Source: CAD feature listing. Evaluate the final solid. Frame: model axes, mm. Coordinates: 2 decimals unless noted, no trailing zeros. Write each loop counter-clockwise with the first axis right and the second up, starting at its lowest first coordinate (ties: lowest second). Pieces come first, ordered by that corner, then holes. Notation, with made-up numbers: M -34,-12.5 L 8,-12.5 A34 cw 8,24.5 Z; hole C -29.75,82 d10. An arc over 180 degrees is marked long. One line per item, written item: value. Start each with the question number.
Item 1: Pin query (flat end, axial travel): P1, Ø8, axis at y = -8, z = 13.5, coming from the -X side; P2, Ø4, axis at x = 11.5, y = 9.5, coming from the +Z side; P3, Ø4, axis at y = 0, z = 33.5, coming from the +X side. Return the tip coordinate at first contact, or that it passes through.
Item 2: Cut plane A-A, the plane y = -1. Output: boundary loops of the cut face in (x, z) (1 decimal).
Item 3: Ray query, L1, parallel to Z at x = 35.5, y = 5; L2, parallel to X at y = -0.5, z = -10; L3, parallel to X at y = -11, z = 29. Return the intervals inside material, ascending. Write a range as from..to.
Item 4: Cut plane B-B, the plane y = 13.5. Output: boundary loops of the cut face in (x, z) (1 decimal), then the cut area to 3 significant figures.
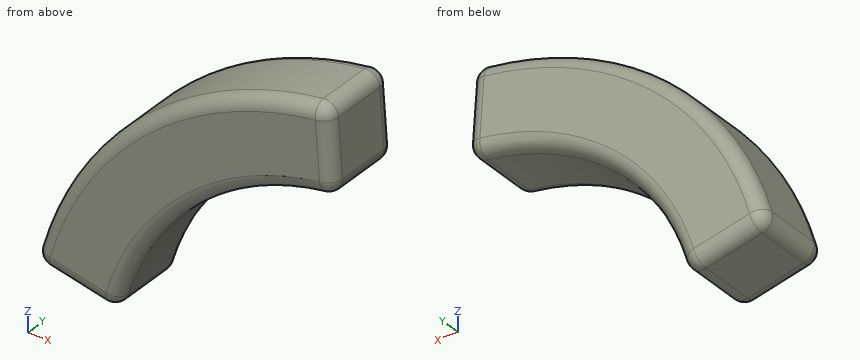
```python
from build123d import *

# Parameters (mm, degrees)
F1_DEPTH = 15.875
F2_R     = 5.08


with BuildPart() as f1:
    # F0 (on Front) → F1 (new body, symmetric)
    with BuildSketch(Plane.XZ):
        with BuildLine():
            ThreePointArc((-24.109727, -54.845564), (5.564563, -6.703762), (57.928178, 14.656209))
            Line((57.928178, 14.656209), (55.651654, 46.32449))
            ThreePointArc((55.651654, 46.32449), (-14.958741, 17.521359), (-54.973422, -47.396077))
            Line((-54.973422, -47.396077), (-24.109727, -54.845564))
        make_face()
    extrude(amount=F1_DEPTH, both=True)

    # F2
    f2_edges = [f1.edges().sort_by_distance(p)[0] for p in [
        (-14.958741, -15.875, 17.521359),
        (5.564563, -15.875, -6.703762),
        (57.928178, 0, 14.656209),
        (56.789916, 15.875, 30.490349),
        (55.651654, 0, 46.32449),
        (56.789916, -15.875, 30.490349),
        (-14.958741, 15.875, 17.521359),
        (5.564563, 15.875, -6.703762),
        (-24.109727, 0, -54.845564),
        (-39.541574, 15.875, -51.12082),
        (-54.973422, 0, -47.396077),
        (-39.541574, -15.875, -51.12082),
    ]]
    fillet(f2_edges, radius=F2_R)


solid = f1.part
```
From the geometry:
1. P1: stops at x = -23.56
1. P2: stops at z = 35.57
1. P3: stops at x = 56.72
2. outline: M -53.6,-42.3 A5.1 ccw -49.9,-48.6 L -28.9,-53.7 A5.1 ccw -22.9,-50.2 A91.1 cw 53.1,14.2 A5.1 ccw 57.6,19.6 L 56,41.1 A5.1 ccw 50.4,45.8 A122.9 ccw Z
3. L1: z = 10.17..43.18
3. L2: x = -39.03..1.88
3. L3: x = 1.04..56.89
4. outline: M -52.9,-42.5 A4.3 ccw -49.7,-47.9 L -28.7,-52.9 A4.3 ccw -23.6,-50 A91.9 cw 53,15 A4.3 ccw 56.8,19.5 L 55.2,41.1 A4.3 ccw 50.5,45.1 A122.1 ccw Z
4. area: 4,010 mm²
